Geometry: see drawing. Coordinates: mm, zero at the bounding-box minimum. A direction names the side the tool comes from. Coordinates: 2 decimals unless noted, no trailing zeros. Order: outer loops, then holes, each group sorted by start corner. A loop starts at its lowest first (then second) coordinate and runs counter-clockwise, first axis right, second up.
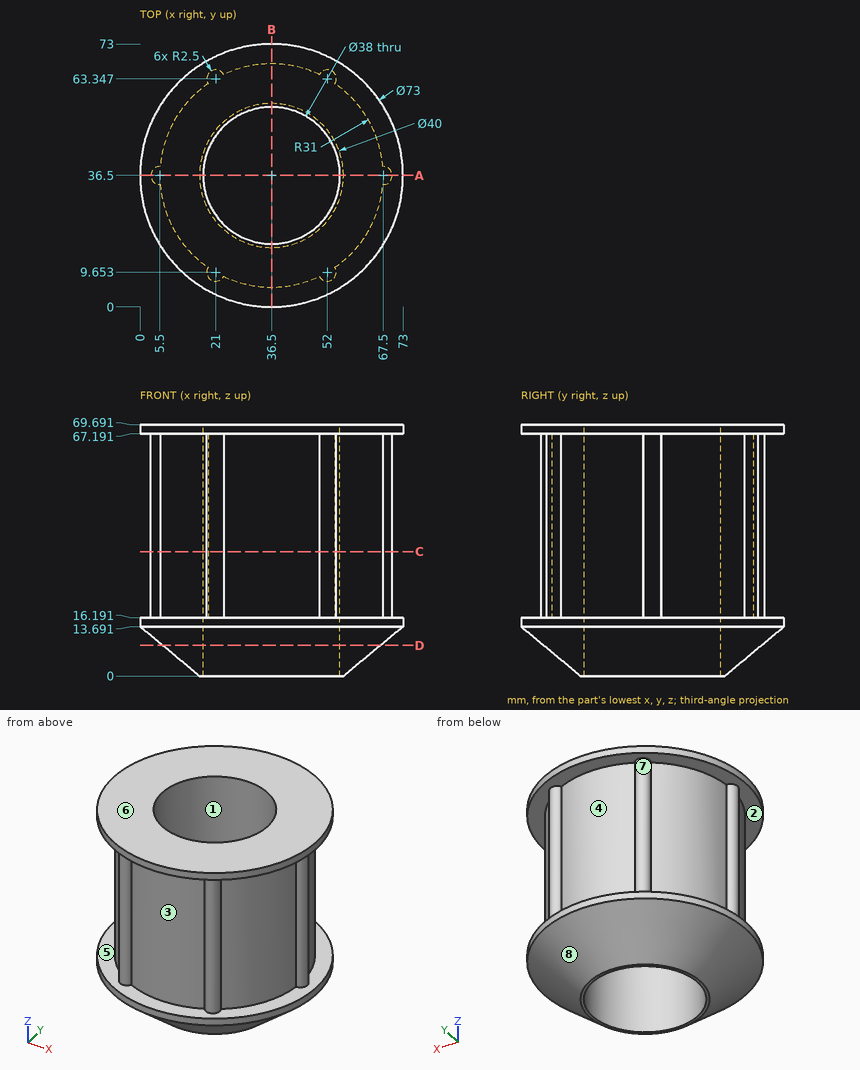
Q1. Section query B-B on x = 36.5. Output: boundary loops of the cut face in (y, z).
Solutions:
outline: (0, 13.69) - (16.5, 0) - (17.5, 0) - (17.5, 69.69) - (0, 69.69) - (0, 67.19) - (5.5, 67.19) - (5.5, 16.19) - (0, 16.19) - close; (55.5, 0) - (56.5, 0) - (73, 13.69) - (73, 16.19) - (67.5, 16.19) - (67.5, 67.19) - (73, 67.19) - (73, 69.69) - (55.5, 69.69) - close
Q2. Section query C-C on z = 34.5. Output: boundary loops of the cut face in (x, y), plus the area to 4 significant figures.
Solutions:
outline: (5.6, 34) arc R31 ccw to (18.89, 10.99) arc R2.5 ccw (long way) to (23.21, 8.49) arc R31 ccw to (49.79, 8.49) arc R2.5 ccw (long way) to (54.11, 10.99) arc R31 ccw to (67.4, 34) arc R2.5 ccw (long way) to (67.4, 39) arc R31 ccw to (54.11, 62.01) arc R2.5 ccw (long way) to (49.79, 64.51) arc R31 ccw to (23.21, 64.51) arc R2.5 ccw (long way) to (18.89, 62.01) arc R31 ccw to (5.6, 39) arc R2.5 ccw (long way) to start; hole circle Ø38 at (36.5, 36.5)
area: 1,945 mm2
Q3. Section query A-A on y = 36.5. Output: boundary loops of the cut face in (x, z).
Solutions:
outline: (0, 13.69) - (16.5, 0) - (17.5, 0) - (17.5, 69.69) - (0, 69.69) - (0, 67.19) - (3, 67.19) - (3, 16.19) - (0, 16.19) - close; (55.5, 0) - (56.5, 0) - (73, 13.69) - (73, 16.19) - (70, 16.19) - (70, 67.19) - (73, 67.19) - (73, 69.69) - (55.5, 69.69) - close
Q4. Pin query (flat end, axial travel): P1, Ø2, axis at y = 51.5, z = 13, coming from the -X side; P2, Ø10, axis at x = 31.5, z = 28, coming from the +Y side; P3, Ø6, axis at y = 24, z = 39.5, coming from the +X side. Return the tip coordinate at first contact, or that it passes through.
Solutions:
P1: stops at x = 2.91
P2: stops at y = 67.5
P3: stops at x = 66.01
Q5. Section query D-D on z = 8.5. Output: boundary loops of the cut face in (x, y), plus the area to 3 significant figures.
Solutions:
outline: circle Ø60.49 at (36.5, 36.5); hole circle Ø38 at (36.5, 36.5)
area: 1,740 mm2
Q6. Set-up query: the marked faces 1, 2, 3 and 4. Return all of +Z, -Z, +X, -X, +Y, -Y with unobstructed straight access to the full face (end or side cutting, diameter ignored); none if empty.
Solutions:
face 1: +Z, -Z
face 2: none
face 3: -Y
face 4: +Y
Q7. Material intervals for line 1 along Y through (x, z) = (36, 38) (1 decimal); line 2 along Y through (x, z) = (47.5, 54) (1 decimal); line 3 along Z through (x, y) = (65, 18.5) (1 decimal), sorted ascending.
Solutions:
line 1: y = 5.5 to 17.5, 55.5 to 67.5
line 2: y = 7.5 to 21, 52 to 65.5
line 3: z = 11.4 to 16.2, 67.2 to 69.7
Q8. Pull-direction query (Z, two-part tool) for the marked faces 5, 6, 7 and 8; classes: pulls with the +Z half, pulls with the -Z half, needs draft (parallel to the pull), parting line crosses it, or undercut.
Solutions:
face 5: undercut
face 6: pulls with the +Z half
face 7: undercut
face 8: pulls with the -Z half
